Input: part model. Units: mm. Frame: model coordinates. A direction names the side the tool comes from. Give positions to 0.01 mm unless a question says otherwise; leave off trailing zeros. Loops run counter-clockwise (first coordinate to the right, second up) from the corner with the lowest first, then second, coordinate; pieces in that order, holes last. Notation, with made-up numbers: (-7.75, 10.5) -> (24.25, 10.5) arc R21 ccw to (24.25, 46.5) -> close; hole circle Ø11 at (49, 74). An arc over 180 degrees is marked (long way). Answer as a JSON object with one key per item and string values.
```python
from build123d import *
from build123d.topology import SkipClean

# Parameters (mm, degrees)
SKETCH_1_W          = 20
SKETCH_1_H          = 37.497986241
CUT_EXTRUDE_START   = -30
CUT_EXTRUDE_1_DEPTH = 52.5


with BuildPart() as part:
    # Sketch 1 → Revolve 3 (revolve)
    with SkipClean():  # the faces are left unmerged after this step: merging them gives an invalid solid
        with BuildSketch(Plane.XY, mode=Mode.PRIVATE) as revolve_3_sk:
            with BuildLine():
                Line((0, 0), (25, 0))
                Line((25, 0), (25, 37.497986241))
                ThreePointArc((25, 37.497986241), (14.577379737, 26.535686679), (0, 22.497986241))
                Line((0, 22.497986241), (0, 0))
            make_face()
            with Locations((35, 18.74899312)):
                Rectangle(SKETCH_1_W, SKETCH_1_H)
            with BuildLine():
                Line((45, 0), (45, -37.497986241))
                ThreePointArc((45, -37.497986241), (71.515080352, -26.515080352), (82.497986241, 0))
                Line((82.497986241, 0), (45, 0))
            make_face()
            with BuildLine():
                Line((45, 37.497986241), (45, 0))
                Line((45, 0), (82.497986241, 0))
                ThreePointArc((82.497986241, 0), (71.515080352, 26.515080352), (45, 37.497986241))
            make_face()
        revolve_3 = revolve(revolve_3_sk.sketch.rotate(Axis((82.497986241, 0, 0), (1, 0, 0)), 90), axis=Axis((82.497986241, 0, 0), (1, 0, 0)))
    add(part.part.scale(1), mode=Mode.REPLACE)  # the faces are merged on a copy

    # Sketch 2 → Cut-Extrude 1 (cut)
    with BuildSketch(Plane.ZY.offset(CUT_EXTRUDE_START)):
        with BuildLine():
            Line((-10, 36.139991314), (-10, 20))
            ThreePointArc((-10, 20), (-12.928932188, 12.928932188), (-20, 10))
            Line((-20, 10), (-36.139991314, 10))
            ThreePointArc((-36.139991314, 10), (-26.515080352, 26.515080352), (-10, 36.139991314))
        make_face()
        with BuildLine():
            Line((36.139991314, 10), (20, 10))
            ThreePointArc((20, 10), (12.928932188, 12.928932188), (10, 20))
            Line((10, 20), (10, 36.139991314))
            ThreePointArc((10, 36.139991314), (26.515080352, 26.515080352), (36.139991314, 10))
        make_face()
        with BuildLine():
            Line((10, -36.139991314), (10, -20))
            ThreePointArc((10, -20), (12.928932188, -12.928932188), (20, -10))
            Line((20, -10), (36.139991314, -10))
            ThreePointArc((36.139991314, -10), (26.515080352, -26.515080352), (10, -36.139991314))
        make_face()
        with BuildLine():
            Line((-36.139991314, -10), (-20, -10))
            ThreePointArc((-20, -10), (-12.928932188, -12.928932188), (-10, -20))
            Line((-10, -20), (-10, -36.139991314))
            ThreePointArc((-10, -36.139991314), (-26.515080352, -26.515080352), (-36.139991314, -10))
        make_face()
    cut_extrude_1 = extrude(amount=-CUT_EXTRUDE_1_DEPTH, mode=Mode.SUBTRACT)

    # Mirror 1: Revolve 3, Cut-Extrude 1 across plane
    with SkipClean():  # the faces are left unmerged after this step: merging them gives an invalid solid
        add(revolve_3.mirror(Plane(origin=(0, 0, 0), x_dir=(0, 0, 1), z_dir=(1, 0, 0))))
        add(cut_extrude_1.mirror(Plane(origin=(0, 0, 0), x_dir=(0, 0, 1), z_dir=(1, 0, 0))), mode=Mode.SUBTRACT)
    add(part.part.scale(1), mode=Mode.REPLACE)  # the faces are merged on a copy


solid = part.part
```
Q1. Section A-A, the plane x = -22. Return the cut outline in (y, z), then the cut area to 3 significant figures.
Evaluation:
{"outline": "circle Ø65.95 at (0, 0)", "area": "3,420 mm2"}
Q2. Pin query (flat end, axial travel): pin 1 (8 mm diameter, centred on x = 59, z = -29.5, fed in from +Y); pin 2 (12 mm diameter, centred on x = 42, y = -27, fed in from -Z); pin 3 (1.5 mm diameter, centred on x = -6, z = 5, fed in from -Y). Return the tip coordinate at first contact, or that it passes through.
Evaluation:
{"pin 1": "stops at y = 10", "pin 2": "stops at z = -10", "pin 3": "stops at y = -22.83"}
Q3. Section B-B, the plane x = 16.5. Return the cut outline in (y, z), then the cut area to 3 significant figures.
Evaluation:
{"outline": "circle Ø55.6 at (0, 0)", "area": "2,430 mm2"}
Q4. Draft query along X for faces 4 (the flat face through (30, -20, -20)), 5 (the cylindrical face through (53.53, -13.01, 12.85)), 6 (the flat face through (-30, 20, 20)). Return one class per face: +X half, -X half, draft (parallel to the pull), parting line (faces both ways), or undercut.
Evaluation:
{"face 4": "+X half", "face 5": "draft", "face 6": "-X half"}
Q5. Ray query, line 1 along X through (y, z) = (21, 31); line 2 along Z through (x, y) = (33.5, -0.5); line 3 along Y through (x, z) = (31.5, 32.5). Return the intervals inside material, ascending.
Evaluation:
{"line 1": "x = -30 to -24.97, 24.97 to 30", "line 2": "z = -37.49 to 37.49", "line 3": "y = -10 to 10"}
Q6. Access query for faces 1 (the flat face through (-47, -10, 28)), 2 (the flat face through (47, 28, -10)), 3 (the flat face through (47, -28, -10)). Directions: +Z, -Z, +X, -X, +Y, -Y. A direction counts if a zero-diameter tool reaches every point of the face in a straight line with its end or side. Return the directions, or none.
Evaluation:
{"face 1": "+Z, -X, -Y", "face 2": "-Z, +X, +Y", "face 3": "-Z, +X, -Y"}
